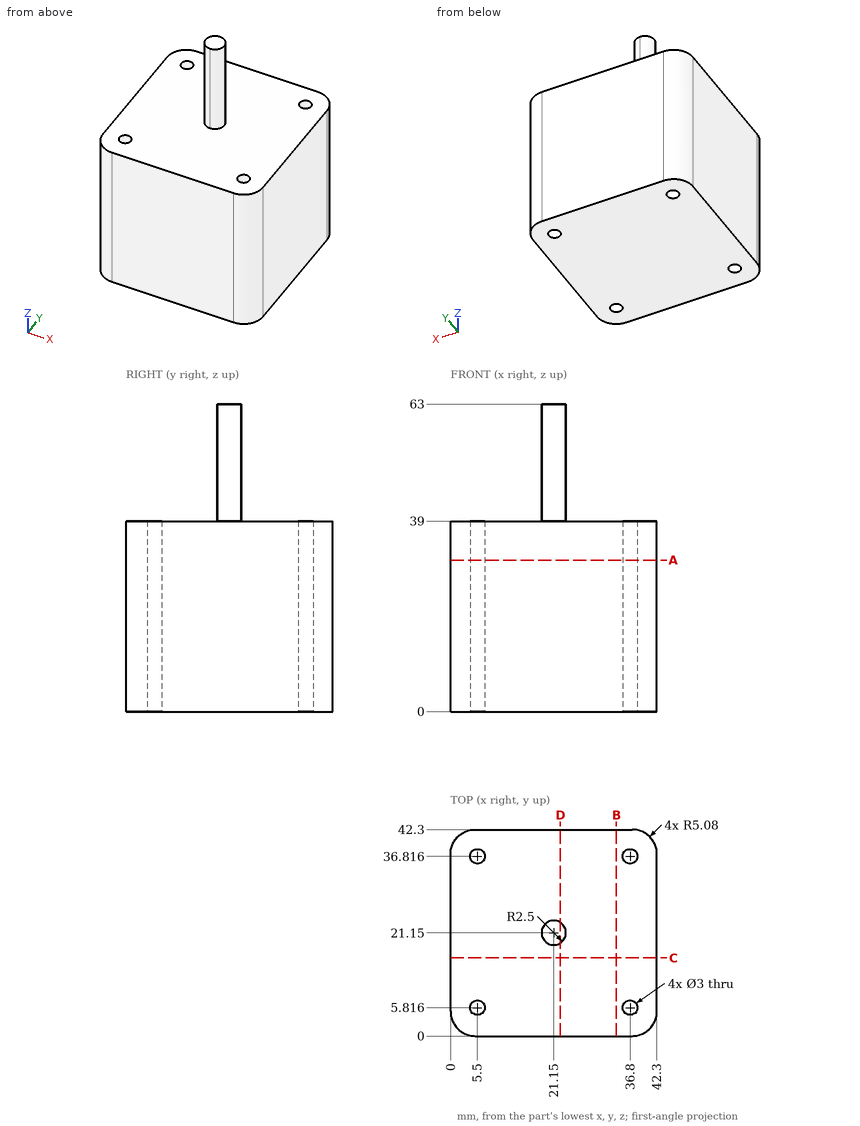
Study the drawing (mm; zero at the part's minimum x, y, z) and answer. Round coordinates to 2 decimals unless told otherwise and drop trailing zeros. Loops run counter-clockwise (first coordinate to the right, second up) from the corner with the lowest first, then second, coordinate; pieces in that order, holes last.
Q1. Given pin 1 Ø5 at (x, y) = (5.5, 36.82) entering from +Z; pin 2 Ø4 at (x, y) = (5.5, 5.82) entering from -Z; pin 3 Ø6 at (x, z) = (35.5, 43) entering from +Y, each flat-ended and moving along its own axis, determine where each tip first touches the part or whether it passes through.
Q2. Section B-B, the plane x = 34 is taken. Determine the outline of the cut face in (y, z), then the cut area to 3 significant figures.
Q3. Section D-D, the plane x = 22.5 is taken. Determine the outline of the cut face in (y, z).
Q4. Section A-A, the plane z = 31 is taken. Determine the outline of the cut face in (x, y).
Q5. Find the intervals of material crossed by line 1 (Y direction, x = 36.8, z = 29); line 2 (X direction, y = 5, z = 37.5); line 3 (Z direction, x = 3, y = 26), in increasing order.
Completed:
1. pin 1: stops at z = 39
1. pin 2: stops at z = 0
1. pin 3: passes through
2. outline: (0, 0) - (42.3, 0) - (42.3, 39) - (0, 39) - close
2. area: 1,650 mm2
3. outline: (0, 0) - (42.3, 0) - (42.3, 39) - (23.25, 39) - (23.25, 63) - (19.05, 63) - (19.05, 39) - (0, 39) - close
4. outline: (0, 5.08) arc R5.08 ccw to (5.08, 0) - (37.22, 0) arc R5.08 ccw to (42.3, 5.08) - (42.3, 37.22) arc R5.08 ccw to (37.22, 42.3) - (5.08, 42.3) arc R5.08 ccw to (0, 37.22) - close; hole circle Ø3 at (5.5, 5.82); hole circle Ø3 at (5.5, 36.82); hole circle Ø3 at (36.8, 5.82); hole circle Ø3 at (36.8, 36.82)
5. line 1: y = 0 to 4.32, 7.32 to 35.32, 38.32 to 42.3
5. line 2: x = 0 to 4.24, 6.76 to 35.54, 38.06 to 42.3
5. line 3: z = 0 to 39
